The listing builds one solid part. Answer for the finished solid, in the listing's coordinates (mm). A direction names the side the tool comes from. Coordinates: 2 decimals unless noted, no trailing zeros. Write each loop counter-clockwise with the first axis right and the second up, starting at its lowest first coordinate (ties: lowest second). Pieces come first, ordered by that corner, then holes.
(1) The part is cut by section C-C on z = 15.5. Determine the outline of the cut face in (x, y).
(2) Given P1, Ø3, axis at x = 0, z = 15.5, coming from the -Y side; P2, Ø7, axis at x = 0, y = 0, coming from the -Z side; P3, Ø3, axis at x = -14, y = 10.5, coming from the +Z side; P4, Ø10, axis at y = 14, z = 10, coming from the -X side, each flat-ended and moving along its own axis, determine where each tip first touches the part or whether it passes through.
(3) The part is cut by section D-D on x = 9. Determine the outline of the cut face in (y, z).
(4) For a pull along Z with two mould halves and no side action, classify faces 1 (the cylindrical face through (8.98, 2.48, 15.17)), 2 (the flat face through (12, -12, 11)), 3 (the cylindrical face through (-5.47, -24.65, 5.45)), 4 (the cylindrical face through (-21.625, -16.581, 10.113)) as +Z half, -Z half, draft (parallel to the pull), parting line (faces both ways), or undercut.
(5) Straight lines are drawn through the part: line 1 (Z direction, x = 7, y = 0); line 2 (Y direction, x = 0, z = 11.5); line 3 (Y direction, x = 0, z = 5.5). For each, find the intervals that lie inside material, in ascending order.
(6) Which of the six approach directions +Z, -Z, +X, -X, +Y, -Y give full straight-line access (tool end or side, diameter ignored) to faces 5 (the flat face through (18, -18, 9.25)), 6 (the cylindrical face through (-3.252, -14.643, 15.437)), 7 (the cylindrical face through (0, 9, 18))?
(7) The part is cut by section A-A on x = 0. Determine the outline of the cut face in (y, z).
from build123d import *

# Parameters (mm, degrees)
SKETCH1_R               = 27.25
BOSS_EXTRUDE1_DEPTH     = 1.75
SKETCH2_R               = 25.25
BOSS_EXTRUDE2_DEPTH     = 7.5
SKETCH3_R               = 27.25
BOSS_EXTRUDE3_DEPTH     = 1.75
SKETCH4_R               = 15
BOSS_EXTRUDE4_DEPTH     = 9
SKETCH6_R               = 4
CUT_EXTRUDE1_DEPTH      = 20
CUT_EXTRUDE2_REACH      = 45.418
CUT_EXTRUDE2_END_RADIUS = 15
SKETCH7_R               = 2.5
CUT_EXTRUDE3_REACH      = 45.418
CUT_EXTRUDE3_END_RADIUS = 15
SKETCH8_R               = 2.5


with BuildPart() as part:
    # Sketch1 → Boss-Extrude1 (new body)
    with BuildSketch(Plane.XY):
        Circle(SKETCH1_R)
    extrude(amount=BOSS_EXTRUDE1_DEPTH)

    # Sketch2 → Boss-Extrude2 (add)
    with BuildSketch(Plane.XY.offset(1.75)):
        Circle(SKETCH2_R)
    extrude(amount=BOSS_EXTRUDE2_DEPTH)

    # Sketch3 → Boss-Extrude3 (add)
    with BuildSketch(Plane.XY.offset(9.25)):
        Circle(SKETCH3_R)
    extrude(amount=BOSS_EXTRUDE3_DEPTH)

    # Sketch4 → Boss-Extrude4 (add)
    with BuildSketch(Plane.XY.offset(11)):
        Circle(SKETCH4_R)
    extrude(amount=BOSS_EXTRUDE4_DEPTH)

    # Sketch6 → Cut-Extrude1 (cut)
    with BuildSketch(Plane.XY.offset(20)):
        Circle(SKETCH6_R)
    extrude(amount=-CUT_EXTRUDE1_DEPTH, mode=Mode.SUBTRACT)

    # Cut-Extrude2: up to this cylinder (the profile starts inside it)
    cut_extrude2_end = Plane(origin=(0, 0, 15.5), z_dir=(0, 0, -1)) * Cylinder(CUT_EXTRUDE2_END_RADIUS, 121.836, mode=Mode.PRIVATE)
    # Sketch7 → Cut-Extrude2 (cut, up to the surface)
    with BuildSketch(Plane.ZY, mode=Mode.PRIVATE) as cut_extrude2_sk1:
        with Locations((15.5, 0)):
            Circle(SKETCH7_R)
    cut_extrude2_tool1 = extrude(cut_extrude2_sk1.sketch, amount=-CUT_EXTRUDE2_REACH, mode=Mode.PRIVATE) & cut_extrude2_end
    add(cut_extrude2_tool1.solids().sort_by_distance((0, 0, 15.5))[0], mode=Mode.SUBTRACT)

    # Cut-Extrude3: up to this cylinder (the profile starts inside it)
    cut_extrude3_end = Plane(origin=(0, 0, 15.5), z_dir=(0, 0, -1)) * Cylinder(CUT_EXTRUDE3_END_RADIUS, 121.836, mode=Mode.PRIVATE)
    # Sketch8 → Cut-Extrude3 (cut, up to the surface)
    with BuildSketch(Plane(origin=(0, 0, 0), x_dir=(0, 0, 1), z_dir=(0, -1, 0)), mode=Mode.PRIVATE) as cut_extrude3_sk1:
        with Locations(Location((15.5, 0, 0), (0, 0, 180))):
            Circle(SKETCH8_R)
    cut_extrude3_tool1 = extrude(cut_extrude3_sk1.sketch, amount=-CUT_EXTRUDE3_REACH, mode=Mode.PRIVATE) & cut_extrude3_end
    add(cut_extrude3_tool1.solids().sort_by_distance((0, 0, 15.5))[0], mode=Mode.SUBTRACT)


solid = part.part
Model answer:
1. outline: (-2.5, 3.12) - (-2.5, 14.79) arc R15 ccw (long way) to (14.79, -2.5) - (3.12, -2.5) arc R4 cw (long way) to start; (2.5, 3.12) arc R4 cw to (3.12, 2.5) - (14.79, 2.5) arc R15 ccw to (2.5, 14.79) - close
2. P1: stops at y = -15
2. P2: passes through
2. P3: stops at z = 11
2. P4: stops at x = -25.72
3. outline: (-25.72, 0) - (25.72, 0) - (25.72, 1.75) - (23.59, 1.75) - (23.59, 9.25) - (25.72, 9.25) - (25.72, 11) - (12, 11) - (12, 20) - (-12, 20) - (-12, 11) - (-25.72, 11) - (-25.72, 9.25) - (-23.59, 9.25) - (-23.59, 1.75) - (-25.72, 1.75) - close; hole circle Ø5 at (0, 15.5)
4. face 1: undercut
4. face 2: +Z half
4. face 3: undercut
4. face 4: draft
5. line 1: z = 0 to 13, 18 to 20
5. line 2: y = -15 to -4, 4 to 15
5. line 3: y = -25.25 to -4, 4 to 25.25
6. face 5: none
6. face 6: +Z
6. face 7: +Y
7. outline: (-27.25, 0) - (-4, 0) - (-4, 20) - (-15, 20) - (-15, 11) - (-27.25, 11) - (-27.25, 9.25) - (-25.25, 9.25) - (-25.25, 1.75) - (-27.25, 1.75) - close; (4, 0) - (27.25, 0) - (27.25, 1.75) - (25.25, 1.75) - (25.25, 9.25) - (27.25, 9.25) - (27.25, 11) - (15, 11) - (15, 13) - (4, 13) - close; (4, 18) - (15, 18) - (15, 20) - (4, 20) - close
